from build123d import *

# Parameters (mm, degrees)
SKETCH_1_R          = 5.5
EXTRUDE_1_DEPTH     = 5
SKETCH_2_R          = 7.25
EXTRUDE_2_DEPTH     = 16
CUT_EXTRUDE_1_DEPTH = 13.5
SKETCH_4_R          = 3.025
CUT_EXTRUDE_2_DEPTH = 6.5
SKETCH_5_R          = 3.525
CUT_EXTRUDE_3_DEPTH = 4.5


with BuildPart() as part:
    # Sketch 1 → Extrude 1 (new body)
    with BuildSketch(Plane(origin=(0, 0, 0), x_dir=(1, 0, 0), z_dir=(0, 1, 0))):
        with Locations(Location((0, 0, 0), (0, 0, 270))):
            Circle(SKETCH_1_R)
    extrude(amount=EXTRUDE_1_DEPTH)

    # Sketch 2 → Extrude 2 (add)
    with BuildSketch(Plane(origin=(0, 0, 0), x_dir=(1, 0, 0), z_dir=(0, 1, 0))):
        with Locations(Location((0, 0, 0), (0, 0, 270))):
            Circle(SKETCH_2_R)
    extrude(amount=-EXTRUDE_2_DEPTH)

    # Sketch 3 → Cut-Extrude 1 (cut)
    with BuildSketch(Plane.XZ.offset(16)):
        with BuildLine():
            Line((2.626904071, 1.5), (-2.626904071, 1.5))
            ThreePointArc((-2.626904071, 1.5), (-0.775963976, -2.923782637), (3.025, 0))
            ThreePointArc((3.025, 0), (2.923782637, 0.775963976), (2.626904071, 1.5))
        make_face()
    extrude(amount=-CUT_EXTRUDE_1_DEPTH, mode=Mode.SUBTRACT)

    # Sketch 4 → Cut-Extrude 2 (cut)
    with BuildSketch(Plane.XZ.offset(16)):
        with Locations(Location((0, 0, 0), (0, 0, 270))):
            Circle(SKETCH_4_R)
    extrude(amount=-CUT_EXTRUDE_2_DEPTH, mode=Mode.SUBTRACT)

    # Sketch 5 → Cut-Extrude 3 (cut)
    with BuildSketch(Plane.XZ.offset(16)):
        with Locations(Location((0, 0, 0), (0, 0, 270))):
            Circle(SKETCH_5_R)
    extrude(amount=-CUT_EXTRUDE_3_DEPTH, mode=Mode.SUBTRACT)


solid = part.part
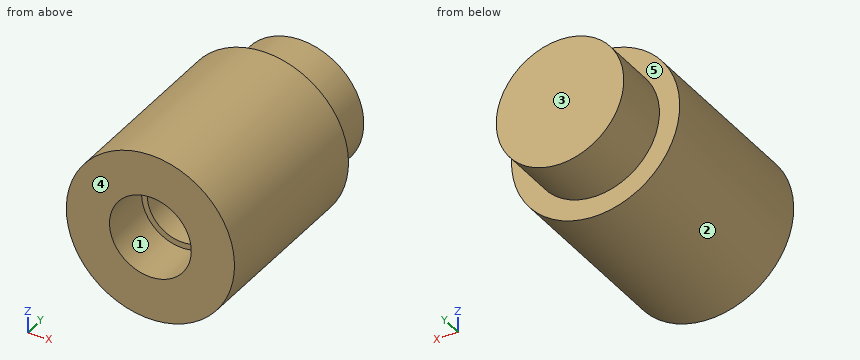
Design review of the part built by this model. Coordinates are the model's own, in mm. Face numbers are marked on the shaded views. A direction names the side the tool comes from. Coordinates: 2 decimals unless noted, no trailing zeros. Write each loop counter-clockwise with the first axis right and the second up, starting at its lowest first coordinate (ties: lowest second). Pieces come first, ordered by that corner, then holes. Notation, with made-up numbers: (-33.75, 75.5) - (-21.75, 75.5) arc R21 ccw to (-21.75, 92.5) - close; hole circle Ø5 at (11, -25). An arc over 180 degrees is marked (long way). One line per item, written item: value.
1) For the marked faces 4 and 5, list the 3-axis set-ups (+Z, -Z, +X, -X, +Y, -Y) from which the entire face can be reached by the end or side of a thin tool; tool diameter is ignored.
Answer sheet:
face 4: +Z, -Z, +X, -X, -Y
face 5: +Y
2) Mouldability with a two-part tool opening along X and no side actions: class the marked faces 1, 2 and 3 as +X half, -X half, draft (parallel to the pull), parting line (faces both ways), or undercut.
Answer sheet:
face 1: undercut
face 2: parting line
face 3: draft
3) Add section C-C (y = 3.25). State the section outline as (x, z) points.
Answer sheet:
outline: circle Ø11 at (0, 0)
4) Add section B-B (x = 0). State the section outline as (y, z) points (3 decimals), plus the area to 4 significant figures.
Answer sheet:
outline: (-16, -7.25) - (0, -7.25) - (0, -5.5) - (5, -5.5) - (5, 5.5) - (0, 5.5) - (0, 7.25) - (-16, 7.25) - (-16, 3.525) - (-11.5, 3.525) - (-11.5, 3.025) - (-9.5, 3.025) - (-9.5, 1.5) - (-2.5, 1.5) - (-2.5, -3.025) - (-11.5, -3.025) - (-11.5, -3.525) - (-16, -3.525) - close
area: 211.5 mm2
5) To check wall thickness, follow probe 1 along X at (y, z) = (-13.9, 0) (3 decimals); probe 2 along X at (y, z) = (-9.25, 0) (3 decimals); probe 3 along Y at (x, z) = (5, 3.75). State the ranges of each line that lie inside material, in increasing order.
Answer sheet:
probe 1: x = -7.25 to -3.525, 3.525 to 7.25
probe 2: x = -7.25 to -3.025, 3.025 to 7.25
probe 3: y = -16 to 0
6) Insertion check: pin 1 (1 mm diameter, centred on x = -4.5, y = -10, fed in from -Z); pin 2 (5 mm diameter, centred on x = 2, z = -1, fed in from -Y); pin 3 (1.4 mm diameter, centred on x = 0, z = 0, fed in from -Y); pin 4 (8 mm diameter, centred on y = -8.5, z = -4.5, fed in from -X). Each pin has a flat end and moves straight along its axis. Give the tip position at first contact, or say it passes through.
Answer sheet:
pin 1: stops at z = -6.05
pin 2: stops at y = -16
pin 3: stops at y = -2.5
pin 4: stops at x = -7.23
7) Add section A-A (y = -4.25). State the section outline as (x, z) points (3 decimals).
Answer sheet:
outline: circle Ø14.5 at (0, 0); hole (-2.627, 1.5) arc R3.025 ccw (long way) to (2.627, 1.5) - close
8) Add section D-D (y = -12.75). State the section outline as (x, z) points (3 decimals), plus the area to 3 significant figures.
Answer sheet:
outline: circle Ø14.5 at (0, 0); hole circle Ø7.05 at (0, 0)
area: 126 mm2
